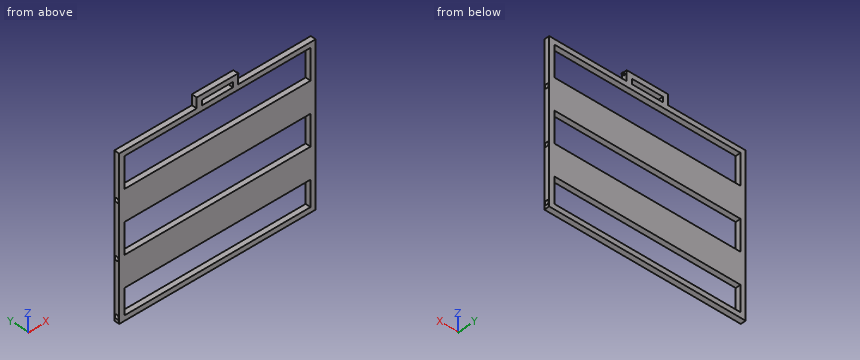
from build123d import *

# Parameters (mm, degrees)
CROQUIS1_W              = 150
CROQUIS1_H              = 25
CROQUIS1_W_2            = 900
CROQUIS1_H_2            = 150
SALIENTE_EXTRUIR1_DEPTH = 25
SALIENTE_EXTRUIR2_DEPTH = 10
SALIENTE_EXTRUIR3_REACH = 927
CROQUIS3_W              = 25
CROQUIS3_H              = 25
CROQUIS4_W              = 25
CROQUIS4_H              = 25
CORTAR_EXTRUIR1_DEPTH   = 951
CROQUIS5_R              = 10
CORTAR_EXTRUIR2_DEPTH   = 20


with BuildPart() as part:
    # Croquis1 → Saliente-Extruir1 (new body)
    with BuildSketch(Plane(origin=(0, 0, 0), x_dir=(1, 0, 0), z_dir=(0, 1, 0))):
        Polygon((-100, -450), (100, -450), (100, -400), (475, -400), (475, 400), (-475, 400), (-475, -400), (-100, -400), align=None)
        with Locations((0, -412.5)):
            Rectangle(CROQUIS1_W, CROQUIS1_H, mode=Mode.SUBTRACT)
        with Locations((0, -300)):
            Rectangle(CROQUIS1_W_2, CROQUIS1_H_2, mode=Mode.SUBTRACT)
        Rectangle(CROQUIS1_W_2, CROQUIS1_H_2, mode=Mode.SUBTRACT)
        with Locations((0, 300)):
            Rectangle(CROQUIS1_W_2, CROQUIS1_H_2, mode=Mode.SUBTRACT)
    extrude(amount=SALIENTE_EXTRUIR1_DEPTH)

    # Croquis2 → Saliente-Extruir2 (add)
    with BuildSketch(Plane(origin=(100, 0, 0), x_dir=(0, 0, -1), z_dir=(1, 0, 0))):
        with BuildLine():
            ThreePointArc((-433.75, 12.5), (-436.064937129, 15.964548247), (-440.151650429, 15.151650429))
            Line((-440.151650429, 15.151650429), (-434.848349571, 9.848349571))
            ThreePointArc((-434.848349571, 9.848349571), (-434.035451753, 11.064937129), (-433.75, 12.5))
        make_face()
        with BuildLine():
            Line((-434.848349571, 9.848349571), (-440.151650429, 15.151650429))
            ThreePointArc((-440.151650429, 15.151650429), (-440.151650429, 9.848349571), (-434.848349571, 9.848349571))
        make_face()
    extrude(amount=SALIENTE_EXTRUIR2_DEPTH)

    # Croquis3 → Saliente-Extruir3 (add, up to next)
    with BuildSketch(Plane(origin=(-450, 0, 0), x_dir=(0, 0, -1), z_dir=(1, 0, 0)), mode=Mode.PRIVATE) as saliente_extruir3_sk1:
        with Locations((362.5, 12.5)):
            Rectangle(CROQUIS3_W, CROQUIS3_H)
    saliente_extruir3_tool1 = extrude(saliente_extruir3_sk1.sketch, amount=SALIENTE_EXTRUIR3_REACH, mode=Mode.PRIVATE) - part.part
    add(saliente_extruir3_tool1.solids().sort_by_distance((-450, 12.5, -362.5))[0])

    # Croquis4 → Cortar-Extruir1 (cut, through all)
    with BuildSketch(Plane.ZY.offset(475)):
        with Locations((-387.5, 12.5)):
            Rectangle(CROQUIS4_W, CROQUIS4_H)
    extrude(amount=-CORTAR_EXTRUIR1_DEPTH, mode=Mode.SUBTRACT)

    # Croquis5 → Cortar-Extruir2 (cut)
    with BuildSketch(Plane(origin=(475, 0, 0), x_dir=(0, 0, -1), z_dir=(1, 0, 0))):
        with Locations((350, 12.5)):
            Circle(CROQUIS5_R)
        with Locations((85, 12.5)):
            Circle(CROQUIS5_R)
        with Locations((-180, 12.5)):
            Circle(CROQUIS5_R)
    cortar_extruir2 = extrude(amount=-CORTAR_EXTRUIR2_DEPTH, mode=Mode.SUBTRACT)

    # Simetría1: Cortar-Extruir2 across plane
    add(cortar_extruir2.mirror(Plane(origin=(-1.209663813, -319.213288435, 1311.891688688), x_dir=(0, 0, 1), z_dir=(1, 0, 0))), mode=Mode.SUBTRACT)


solid = part.part
Model file for the job. Use its own axes, mm. Give positions to 0.01 mm unless a question says otherwise; leave off trailing zeros. Order: outer loops, then holes, each group sorted by start corner. A loop starts at its lowest first (then second) coordinate and runs counter-clockwise, first axis right, second up. Notation, with made-up numbers: (-31, 65) - (5, 65) arc R17 ccw to (5, 77) - close; hole circle Ø11 at (7.25, 67.25). An arc over 180 degrees is marked (long way). Write item = value, one per line. Start each with the question number.
1. Cut at A-A, the plane z = 22. List the corners of the cut face in (x, y).
2. Probe line 1 along Z through (x, y) = (-155, 5.25); line 2 along Z through (x, y) = (-463.5, 12.5); line 3 along Z through (x, y) = (-54, 1.5). List the from-to ranges inside material, lowest first.
3. Drop flat-ended pins along their axis: P1, Ø2, axis at y = 12.5, z = 436, coming from the +X side; P2, Ø10, axis at y = 11, z = -348, coming from the +X side; P3, Ø7.5, axis at y = 13.5, z = 424.5, coming from the -X side. Give the stop position or say it passes through.
4. Cut at B-B, the plane x = -253.5. List the corners of the cut face in (y, z).
Taken from the geometry:
q1.outline = (-475, 0) - (-450, 0) - (-450, 25) - (-475, 25) - close; (450, 0) - (475, 0) - (475, 25) - (450, 25) - close
q2.line_1 = -375 to -350, -225 to -75, 75 to 225, 375 to 400
q2.line_2 = -375 to -360, -340 to -95, -75 to 170, 190 to 400
q2.line_3 = -375 to -350, -225 to -75, 75 to 225, 375 to 400, 425 to 450
q3.P1 = 110
q3.P2 = 455
q3.P3 = -100
q4.outline = (0, -375) - (25, -375) - (25, -350) - (0, -350) - close; (0, -225) - (25, -225) - (25, -75) - (0, -75) - close; (0, 75) - (25, 75) - (25, 225) - (0, 225) - close; (0, 375) - (25, 375) - (25, 400) - (0, 400) - close
